from build123d import *

# Parameters (mm, degrees)
BOSS_EXTRUDE1_DEPTH      = 20
BOSS_EXTRUDE1_DEPTH_BACK = 23
SKETCH5_W                = 30.5
SKETCH5_H                = 37.32
CUT_EXTRUDE1_DEPTH       = 40
SKETCH4_R                = 1.375
SKETCH4_R_2              = 11.5
SKETCH4_R_3              = 6
SKETCH4_R_4              = 3.5
BOSS_EXTRUDE2_DEPTH      = 6.81
SKETCH4_3_R              = 1.375
SKETCH4_3_R_2            = 3.5
CUT_EXTRUDE2_DEPTH       = 6.21
CUT_EXTRUDE2_DEPTH_BACK  = 6.81
CUT_EXTRUDE3_START       = -6.81
SKETCH4_4_R              = 6
SKETCH4_4_R_2            = 3.5
CUT_EXTRUDE3_DEPTH       = 3.5
CUT_EXTRUDE4_START       = 5.21
SKETCH4_5_R              = 11.5
CUT_EXTRUDE4_DEPTH       = 3.5
SKETCH6_R                = 6
CUT_EXTRUDE5_DEPTH       = 1
CUT_EXTRUDE5_DEPTH_BACK  = 39.5000001
CUT_EXTRUDE6_START       = -4
SKETCH6_3_R              = 7
SKETCH6_3_R_2            = 6
CUT_EXTRUDE6_DEPTH       = 1
CUT_EXTRUDE7_START       = -34.5
SKETCH6_4_R              = 7
SKETCH6_4_R_2            = 6
CUT_EXTRUDE7_DEPTH       = 1
SKETCH7_R                = 1.85
SKETCH7_R_2              = 4
CUT_EXTRUDE8_DEPTH       = 4.0000001
SKETCH8_R                = 2.875
CUT_EXTRUDE9_DEPTH       = 5


with BuildPart() as part:
    # Sketch3 → Boss-Extrude1 (new body, two sides)
    with BuildSketch(Plane(origin=(0, 0, 0), x_dir=(1, 0, 0), z_dir=(0, 1, 0))) as boss_extrude1_sk:
        with BuildLine():
            Line((-16.01, 16), (11.49, 16))
            ThreePointArc((11.49, 16), (15.379087297, 14.389087297), (16.99, 10.5))
            Line((16.99, 10.5), (16.99, -25.03))
            ThreePointArc((16.99, -25.03), (15.379087297, -28.919087297), (11.49, -30.53))
            Line((11.49, -30.53), (-16.01, -30.53))
            ThreePointArc((-16.01, -30.53), (-19.899087297, -28.919087297), (-21.51, -25.03))
            Line((-21.51, -25.03), (-21.51, 10.5))
            ThreePointArc((-21.51, 10.5), (-19.899087297, 14.389087297), (-16.01, 16))
        make_face()
    extrude(amount=BOSS_EXTRUDE1_DEPTH)
    extrude(boss_extrude1_sk.sketch, amount=-BOSS_EXTRUDE1_DEPTH_BACK)

    # Sketch5 → Cut-Extrude1 (cut)
    with BuildSketch(Plane(origin=(0, 20, 0), x_dir=(1, 0, 0), z_dir=(0, 1, 0))):
        with Locations((-2.26, -6.66)):
            Rectangle(SKETCH5_W, SKETCH5_H)
    extrude(amount=-CUT_EXTRUDE1_DEPTH, mode=Mode.SUBTRACT)

    # Sketch4 → Boss-Extrude2 (add)
    with BuildSketch(Plane.XY.offset(25.32)):
        with BuildLine():
            ThreePointArc((11.5, 0), (-1.557539449, -11.394036636), (-11.078099281, 3.08637592))
            Line((-11.078099281, 3.08637592), (-17.51, -20))
            Line((-17.51, -20), (12.99, -20))
            Line((12.99, -20), (11.469504194, 0.836942974))
            ThreePointArc((11.469504194, 0.836942974), (11.49237352, 0.41874919), (11.5, 0))
        make_face()
        with Locations((-9.9, -9.9)):
            Circle(SKETCH4_R, mode=Mode.SUBTRACT)
        with Locations((9.9, -9.9)):
            Circle(SKETCH4_R, mode=Mode.SUBTRACT)
        Circle(SKETCH4_R_2)
        with Locations((-9.9, -9.9)):
            Circle(SKETCH4_R)
        with Locations((9.9, -9.9)):
            Circle(SKETCH4_R)
        Circle(SKETCH4_R_3)
        Circle(SKETCH4_R_4, mode=Mode.SUBTRACT)
        Circle(SKETCH4_R_4)
    extrude(amount=-BOSS_EXTRUDE2_DEPTH)

    # Sketch4<3> → Cut-Extrude2 (cut, two sides)
    with BuildSketch(Plane.XY.offset(25.32)) as cut_extrude2_sk:
        with Locations((-9.9, 9.9)):
            Circle(SKETCH4_3_R)
        with Locations((-9.9, -9.9)):
            Circle(SKETCH4_3_R)
        with Locations((9.9, 9.9)):
            Circle(SKETCH4_3_R)
        with Locations((9.9, -9.9)):
            Circle(SKETCH4_3_R)
        Circle(SKETCH4_3_R_2)
    extrude(amount=CUT_EXTRUDE2_DEPTH, mode=Mode.SUBTRACT)
    extrude(cut_extrude2_sk.sketch, amount=-CUT_EXTRUDE2_DEPTH_BACK, mode=Mode.SUBTRACT)

    # Sketch4<4> → Cut-Extrude3 (cut)
    with BuildSketch(Plane.XY.offset(25.32).offset(CUT_EXTRUDE3_START)):
        Circle(SKETCH4_4_R)
        Circle(SKETCH4_4_R_2, mode=Mode.SUBTRACT)
    extrude(amount=CUT_EXTRUDE3_DEPTH, mode=Mode.SUBTRACT)

    # Sketch4<5> → Cut-Extrude4 (cut)
    with BuildSketch(Plane.XY.offset(25.32).offset(CUT_EXTRUDE4_START)):
        Circle(SKETCH4_5_R)
    extrude(amount=-CUT_EXTRUDE4_DEPTH, mode=Mode.SUBTRACT)

    # Sketch6 → Cut-Extrude5 (cut, two sides)
    with BuildSketch(Plane.ZY.offset(21.51)) as cut_extrude5_sk:
        Circle(SKETCH6_R)
    extrude(amount=CUT_EXTRUDE5_DEPTH, mode=Mode.SUBTRACT)
    extrude(cut_extrude5_sk.sketch, amount=-CUT_EXTRUDE5_DEPTH_BACK, mode=Mode.SUBTRACT)

    # Sketch6<3> → Cut-Extrude6 (cut)
    with BuildSketch(Plane.ZY.offset(21.51).offset(CUT_EXTRUDE6_START)):
        Circle(SKETCH6_3_R)
        Circle(SKETCH6_3_R_2, mode=Mode.SUBTRACT)
    extrude(amount=CUT_EXTRUDE6_DEPTH, mode=Mode.SUBTRACT)

    # Sketch6<4> → Cut-Extrude7 (cut)
    with BuildSketch(Plane.ZY.offset(21.51).offset(CUT_EXTRUDE7_START)):
        Circle(SKETCH6_4_R)
        Circle(SKETCH6_4_R_2, mode=Mode.SUBTRACT)
    extrude(amount=-CUT_EXTRUDE7_DEPTH, mode=Mode.SUBTRACT)

    # Sketch7 → Cut-Extrude8 (cut, through all)
    with BuildSketch(Plane(origin=(0, -20, 0), x_dir=(1, 0, 0), z_dir=(0, 1, 0))):
        with Locations((5.656854249, -5.656854249)):
            Circle(SKETCH7_R)
        with Locations((0, -8)):
            Circle(SKETCH7_R)
        with Locations((-5.656854249, -5.656854249)):
            Circle(SKETCH7_R)
        with Locations((-8, 0)):
            Circle(SKETCH7_R)
        with Locations((-5.656854249, 5.656854249)):
            Circle(SKETCH7_R)
        with Locations((0, 8)):
            Circle(SKETCH7_R)
        with Locations((5.656854249, 5.656854249)):
            Circle(SKETCH7_R)
        Circle(SKETCH7_R_2)
        with Locations((8, 0)):
            Circle(SKETCH7_R)
    extrude(amount=-CUT_EXTRUDE8_DEPTH, mode=Mode.SUBTRACT)

    # Sketch8 → Cut-Extrude9 (cut, through all)
    with BuildSketch(Plane.XY.offset(-12)):
        with Locations((-9.9, 9.9)):
            Circle(SKETCH8_R)
        with Locations((9.9, 9.9)):
            Circle(SKETCH8_R)
        with Locations((-9.9, -9.9)):
            Circle(SKETCH8_R)
        with Locations((9.9, -9.9)):
            Circle(SKETCH8_R)
    extrude(amount=-CUT_EXTRUDE9_DEPTH, mode=Mode.SUBTRACT)


solid = part.part
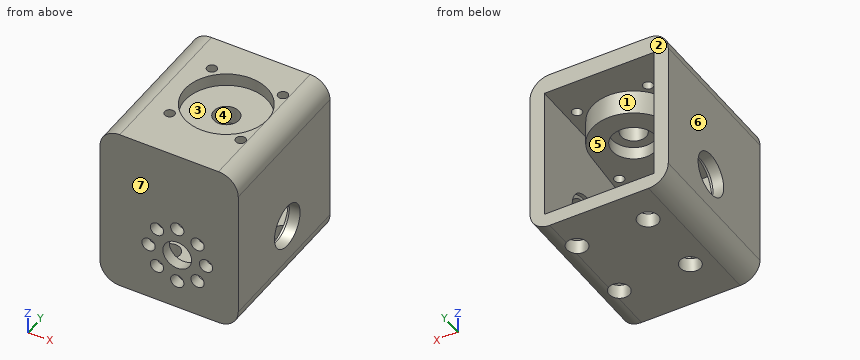
The model under review builds one solid part; all positions refer to its coordinate system, in mm. Face numbers are marked on the shaded views. A direction names the side the tool comes from. Round coordinates to 2 decimals unless told otherwise and drop trailing zeros. Loops run counter-clockwise (first coordinate to the right, second up) from the corner with the lowest first, then second, coordinate; pieces in that order, holes last. Notation, with made-up numbers: (-31, -26) -> (-25, -26) arc R13 ccw to (-25, -13) -> close; hole circle Ø10 at (62, -13.75). An arc over 180 degrees is marked (long way). Answer as CSV lines item,"result".
1) For P1, Ø5, axis at x = 0, z = 8, coming from the -Y side; P2, Ø5, axis at x = 5.66, z = -5.66, coming from the +Y side; P3, Ø4.5, axis at x = -9.9, y = 9.9, coming from the -Z side; P4, Ø9, axis at x = -1.5, y = -3.5, coming from the +Z side, all flat-tipped, find the tip position at first contact; note any pin that passes through.
Geometry results:
P1,"stops at y = -23"
P2,"stops at y = -20"
P3,"stops at z = 25.32"
P4,"stops at z = 27.03"
2) Draft analysis for pull direction X (two halves, no side actions). For the marked faces 4, 5, 6 and 7, state which applies: pulls with the +X half, pulls with the -X half, needs draft (parallel to the pull), parting line crosses it, or undercut.
Geometry results:
face 4,"undercut"
face 5,"undercut"
face 6,"pulls with the -X half"
face 7,"needs draft"
3) Add section A-A on x = 0. State how many separate pieces and enclosed holes the cut face has, plus the area to 3 significant figures.
Geometry results:
separate pieces,"5"
enclosed holes,"0"
area,"519 mm²"
4) To check wall thickness, follow line 1 along X through (y, z) = (-21.3, 0); line 2 along X through (y, z) = (-18, 9.5); line 3 along Z through (x, y) = (6.5, 12.5). State the ranges of each line that lie inside material, in increasing order. Write a range as from..to.
Geometry results:
line 1,"x = -21.51..-9.85, -6.15..-4, 4..6.15, 9.85..16.99"
line 2,"x = -21.51..-17.51, 12.99..16.99"
line 3,"z = -16..-12, 25.32..30.53"
5) Tool access review of the marked faces 1, 2 and 3: name each direction out of +Z, -Z, +X, -X, +Y, -Y from which nothing blocks a thin tool from reaching the whole face with its end or side.
Geometry results:
face 1,"+Y"
face 2,"+Z, -Z, +X, -X, +Y"
face 3,"+Z"
6) Add section B-B on y = 14. Write out the cut boundary in (x, z).
Geometry results:
outline,"(-21.51, -10.5) arc R5.5 ccw to (-16.01, -16) -> (11.49, -16) arc R5.5 ccw to (16.99, -10.5) -> (16.99, 25.03) arc R5.5 ccw to (11.49, 30.53) -> (-16.01, 30.53) arc R5.5 ccw to (-21.51, 25.03) -> close; hole (-17.51, -12) -> (12.99, -12) -> (12.99, 25.32) -> (-17.51, 25.32) -> close"
